```python
from build123d import *

# Parameters (mm, degrees)
F1_DEPTH = 25.4
F2_R     = 11.43
F5_DEPTH = 2.54
F3_R     = 11.43
F6_DEPTH = 2.54
F4_R     = 11.43
F7_DEPTH = 2.54


with BuildPart() as f1:
    # F0 (on Front) → F1 (new body)
    with BuildSketch(Plane.XZ):
        Polygon((38.1075000086, -5.3176727306), (27.9171615839, 26.4781285077), (-3.2953689198, 38.3353589243), (-32.0264194136, 21.3252821721), (-36.6409228691, -11.7431670122), (-13.6640640655, -35.9687719194), (19.6021136755, -33.109157942), align=None)
    extrude(amount=F1_DEPTH)

    # F2 (on face) → F5 (cut)
    with BuildSketch(Plane(origin=(-34.3336711413, 0, 4.7910575799), x_dir=(0, -1, 0), z_dir=(-0.9904036604, 0, 0.1382048819))):
        with Locations((12.7, 0)):
            Circle(F2_R)
    extrude(amount=-F5_DEPTH, mode=Mode.SUBTRACT)

    # F3 (on face) → F6 (cut)
    with BuildSketch(Plane(origin=(-17.6608941667, 0, 29.8303205482), x_dir=(0.8604980965, 0, 0.5094536543), z_dir=(-0.5094536543, 0, 0.8604980965))):
        with Locations((0, -12.7)):
            Circle(F3_R)
    extrude(amount=-F6_DEPTH, mode=Mode.SUBTRACT)

    # F4 (on face) → F7 (cut)
    with BuildSketch(Plane(origin=(12.3108963321, 0, 32.406743716), x_dir=(0.9348186935, 0, -0.3551253445), z_dir=(0.3551253445, 0, 0.9348186935))):
        with Locations((0, -12.7)):
            Circle(F4_R)
    extrude(amount=-F7_DEPTH, mode=Mode.SUBTRACT)


solid = f1.part
```
Model file for the job. Use its own axes, mm. A direction names the side the tool comes from. Coordinates: 2 decimals unless noted, no trailing zeros. Loops run counter-clockwise (first coordinate to the right, second up) from the corner with the lowest first, then second, coordinate; pieces in that order, holes last. Notation, with made-up numbers: (1, -37.5) -> (20, -37.5) arc R8 ccw to (20, -29.5) -> close; hole circle Ø7 at (15.5, -6). An arc over 180 degrees is marked (long way). Answer as a JSON object with one key per item and string values.
Q1. Cut at C-C (z = 19.5). List the corners of the cut face in (x, y), and give its area (3 significant figures).
Report:
{"outline": "(-32.28, -25.4) -> (30.15, -25.4) -> (30.15, 0) -> (-32.28, 0) -> close", "area": "1,590 mm2"}
Q2. Cut at B-B (x = 27). List the corners of the cut face in (y, z).
Report:
{"outline": "(-25.4, -22) -> (0, -22) -> (0, 26.83) -> (-25.4, 26.83) -> close"}
Q3. Flat gauge pins, fed straight in: P1, Ø5, axis at x = -11.5, y = -3.5, coming from the -Z side; P2, Ø2, axis at y = -15.5, z = -4, coming from the +X side; P3, Ø1.5, axis at y = -13, z = 13.5, coming from the +X side; P4, Ø5, axis at x = 21, y = -4, coming from the +Z side. Where does each tip first touch, or does it go through?
Report:
{"P1": "stops at z = -35.97", "P2": "stops at x = 38.01", "P3": "stops at x = 32.32", "P4": "stops at z = 30.03"}
Q4. Pull direction Z, two halves, no side cores. Call faces 1 (the cylindrical face through (-32.62, -23.6, 8.02)), 2 (the flat face through (28.725, -12.522, -19.408)), 3 (the flat face through (0, -25.4, 2)): released by +Z, released by -Z, zero draft, split by the parting line, or undercut.
Report:
{"face 1": "undercut", "face 2": "released by -Z", "face 3": "zero draft"}
Q5. Probe probe 1 along Y at (x, z) = (-21.5, 25); probe 2 along Z at (x, y) = (-16, -22.25); probe 3 along X at (y, z) = (-7.5, 24.5). List the from-to ranges inside material, lowest first.
Report:
{"probe 1": "y = -25.4 to -22.57, -2.83 to 0", "probe 2": "z = -33.51 to 27.86", "probe 3": "x = -26.66 to -26.33, -21.68 to 28.55"}
Q6. Cut at D-D (y = -15.25). List the corners of the cut face in (x, z).
Report:
{"outline": "(-36.64, -11.74) -> (-13.66, -35.97) -> (19.6, -33.11) -> (38.11, -5.32) -> (27.92, 26.48) -> (22.73, 28.45) -> (21.82, 26.08) -> (0.99, 33.99) -> (1.9, 36.36) -> (-3.3, 38.34) -> (-8.07, 35.51) -> (-6.78, 33.32) -> (-25.95, 21.97) -> (-27.25, 24.15) -> (-32.03, 21.33) -> (-32.79, 15.83) -> (-30.28, 15.48) -> (-33.36, -6.59) -> (-35.87, -6.24) -> close"}
Q7. 3-axis set-ups, long thin cutter, end or side, ignore diameter. For faces 4 (the flat face through (-16.505, -12.54, 27.563)), 5 (the flat face through (2.74, -12.52, -34.56)): which of +Z, -Z, +X, -X, +Y, -Y reach the whole face in a straight line?
Report:
{"face 4": "none", "face 5": "-Z, +X, +Y, -Y"}
Q8. Cut at A-A (y = -23). List the corners of the cut face in (x, z).
Report:
{"outline": "(-36.64, -11.74) -> (-13.66, -35.97) -> (19.6, -33.11) -> (38.11, -5.32) -> (27.92, 26.48) -> (16.94, 30.65) -> (16.04, 28.27) -> (6.78, 31.79) -> (7.68, 34.17) -> (-3.3, 38.34) -> (-13.4, 32.35) -> (-12.1, 30.17) -> (-20.63, 25.12) -> (-21.92, 27.31) -> (-32.03, 21.33) -> (-33.65, 9.7) -> (-31.13, 9.35) -> (-32.5, -0.47) -> (-35.02, -0.12) -> close"}
